from build123d import *

# Parameters (mm, degrees)
SKETCH1_W                         = 19.05
SKETCH1_H                         = 25.4
BOSS_EXTRUDE1_DEPTH               = 3.96875
SKETCH2_R                         = 9.921875
CUT_EXTRUDE1_DEPTH                = 24.236683855
SKETCH3_W                         = 7.14375
SKETCH3_H                         = 25.4
CUT_EXTRUDE2_DEPTH                = 24.236683855
SKETCH4_W                         = 6.35
SKETCH4_H                         = 9.525
BOSS_EXTRUDE2_DEPTH               = 7.14375
TAP_DRILL_FOR_2_HELICOIL1_D       = 2.38252
TAP_DRILL_FOR_2_HELICOIL3_D       = 2.38252
TAP_DRILL_FOR_2_HELICOIL3_DEPTH   = 4.7371
TAP_DRILL_FOR_2_HELICOIL3_TIP     = 0.715781221
TAP_DRILL_FOR_2_HELICOIL3_2_D     = 2.38252
TAP_DRILL_FOR_2_HELICOIL3_2_DEPTH = 4.7371
TAP_DRILL_FOR_2_HELICOIL3_2_TIP   = 0.715781221
FILLET1_R                         = 0.79375
FILLET2_RADIUS                    = 3.175
FILLET2_LENGTH                    = 9.525


with BuildPart() as part:
    # Sketch1 → Boss-Extrude1 (new body)
    with BuildSketch(Plane.XY):
        with Locations((9.525, 0)):
            Rectangle(SKETCH1_W, SKETCH1_H)
    extrude(amount=BOSS_EXTRUDE1_DEPTH)

    # Sketch2 → Cut-Extrude1 (cut, through all)
    with BuildSketch(Plane.XY.offset(3.96875)):
        Circle(SKETCH2_R)
    extrude(amount=-CUT_EXTRUDE1_DEPTH, mode=Mode.SUBTRACT)

    # Sketch3 → Cut-Extrude2 (cut, through all)
    with BuildSketch(Plane.XY.offset(3.96875)):
        with Locations((3.571875, 0)):
            Rectangle(SKETCH3_W, SKETCH3_H)
    extrude(amount=-CUT_EXTRUDE2_DEPTH, mode=Mode.SUBTRACT)

    # Sketch4 → Boss-Extrude2 (add)
    with BuildSketch(Plane.XY.offset(3.96875)):
        with Locations((15.875, 0)):
            Rectangle(SKETCH4_W, SKETCH4_H)
    extrude(amount=BOSS_EXTRUDE2_DEPTH)

    # Tap Drill for #2 Helicoil1 (through all)
    with Locations(Plane(origin=(0, 0, 0), x_dir=(-1, 0, 0), z_dir=(0, 0, -1))):
        with Locations((-9.779, 9.779), (-9.779, -9.779), (-15.875, 7.9375), (-15.875, -7.9375)):
            Hole(TAP_DRILL_FOR_2_HELICOIL1_D / 2)

    # Tap Drill for _2 Helicoil3
    with Locations(Plane(origin=(0, 4.7625, 0), x_dir=(1, 0, 0), z_dir=(0, 1, 0))):
        with Locations((15.875, -7.9375)):
            Hole(TAP_DRILL_FOR_2_HELICOIL3_D / 2, depth=TAP_DRILL_FOR_2_HELICOIL3_DEPTH)
            with Locations((0, 0, -(TAP_DRILL_FOR_2_HELICOIL3_DEPTH + TAP_DRILL_FOR_2_HELICOIL3_TIP / 2))):  # 118° drill point
                Cone(0, TAP_DRILL_FOR_2_HELICOIL3_D / 2, TAP_DRILL_FOR_2_HELICOIL3_TIP, mode=Mode.SUBTRACT)

    # Tap Drill for _2 Helicoil3 2
    with Locations(Plane(origin=(0, -4.7625, 0), x_dir=(-1, 0, 0), z_dir=(0, -1, 0))):
        with Locations((-15.875, -7.9375)):
            Hole(TAP_DRILL_FOR_2_HELICOIL3_2_D / 2, depth=TAP_DRILL_FOR_2_HELICOIL3_2_DEPTH)
            with Locations((0, 0, -(TAP_DRILL_FOR_2_HELICOIL3_2_DEPTH + TAP_DRILL_FOR_2_HELICOIL3_2_TIP / 2))):  # 118° drill point
                Cone(0, TAP_DRILL_FOR_2_HELICOIL3_2_D / 2, TAP_DRILL_FOR_2_HELICOIL3_2_TIP, mode=Mode.SUBTRACT)

    # Fillet1
    fillet1_edges = [part.edges().sort_by_distance(p)[0] for p in [
        (12.7, 0, 3.96875),
    ]]
    fillet(fillet1_edges, radius=FILLET1_R)

    # Fillet2: full round fillet: the end face becomes a half cylinder, R = half its width
    fillet2_face = Plane((15.875, 0, 11.1125), x_dir=(0, 1, 0), z_dir=(0, 0, 1))  # on the end face: x along it, z out of the body
    fillet2_slab = fillet2_face.offset(-FILLET2_RADIUS / 2) * Box(FILLET2_LENGTH, 2 * FILLET2_RADIUS, FILLET2_RADIUS, mode=Mode.PRIVATE)  # the body's end, R deep
    fillet2_round = Plane((15.875, 0, 7.9375), x_dir=(0, 0, 1), z_dir=(0, 1, 0)) * Cylinder(FILLET2_RADIUS, FILLET2_LENGTH, mode=Mode.PRIVATE)  # its axis R under the face
    add(fillet2_slab - fillet2_round, mode=Mode.SUBTRACT)


solid = part.part
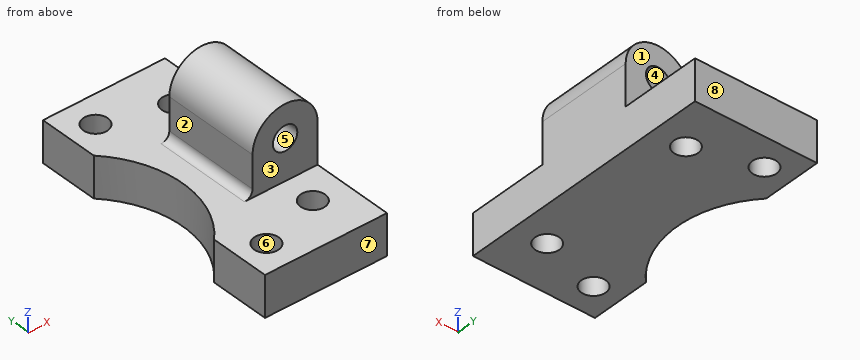
Could you check a few things on this model? Use its own coordinates, in mm. Face numbers are marked on the shaded views. A direction names the side the tool comes from. Coordinates: 2 decimals unless noted, no trailing zeros. Order: outer loops, then holes, each group sorted by start corner. A loop starts at its lowest first (then second) coordinate and runs counter-clockwise, first axis right, second up. Notation, with made-up numbers: (1, 3.25) - (27, 3.25) arc R24 cw to (27, 17.25) - close; hole circle Ø11 at (31.5, 32.5). An arc over 180 degrees is marked (long way). Answer in a Markdown table with one row per item. Add a question column.
(1) I need wall thicknesses on L1, parallel to Y at x = 12.75, z = 4.25; L2, parallel to Z at x = 15.75, y = 4.25; L3, parallel to Z at x = 10.5, y = 8.5. Which ranges of each line are inside material? Lowest first, please.
(2) If we section it at B-B, the plane x = 10.5: Please give me the cut outline in (y, z), then the cut area to 3 significant figures.
(3) Will these pins go through, and if not, where does the flat tip stop? pin 1 (6 mm diameter, centred on x = 12.5, y = 0, fed in from +Z); pin 2 (1.5 mm diameter, centred on y = -4.5, z = 5.5, fed in from -X); pin 3 (2 mm diameter, centred on x = 15.88, y = -7.94, fed in from +Z); pin 4 (2 mm diameter, centred on x = 14.5, z = 7.5, fed in from -Y).
(4) If we mould it in two halves opening along Y, with no side actions, what happens to the marked faces 5, 6, 7 and 8? For each: released by +Y, released by -Y, zero draft, split by the parting line, or undercut.
(5) On a 3-axis mill with a long thin cutter (end or side, diameter ignored), from which of +Z, -Z, +X, -X, +Y, -Y can I reach the whole of each face in a straight line? I mean the marked faces 1, 2, 3 and 4. Say none if no direction works.
(6) If we section it at D-D, the plane z = 3: State how many separate pieces and enclosed holes the cut face has, then the cut area to 3 significant figures.
(7) If we section it at A-A, the plane y = -7.5: Please give me the cut outline in (x, z), then the cut area to 3 significant figures.
Results are:
| question | item | result |
|---|---|---|
| 1 | L1 | y = -4.76 to 4.76 |
| 1 | L2 | z = 0 to 6.75, 9.12 to 11.11 |
| 1 | L3 | z = 0 to 3.97 |
| 2 | outline | (-12.7, 0) - (-10.73, 0) - (-10.73, 3.97) - (-12.7, 3.97) - close; (-8.83, 0) - (8.83, 0) - (8.83, 3.97) - (-8.83, 3.97) - close; (10.73, 0) - (12.7, 0) - (12.7, 3.97) - (10.73, 3.97) - close |
| 2 | area | 85.8 mm2 |
| 3 | pin 1 | stops at z = 11.09 |
| 3 | pin 2 | stops at x = 12.7 |
| 3 | pin 3 | passes through |
| 3 | pin 4 | stops at y = -4.76 |
| 4 | face 5 | zero draft |
| 4 | face 6 | undercut |
| 4 | face 7 | released by -Y |
| 4 | face 8 | released by +Y |
| 5 | face 1 | +Z, +X, -X, +Y |
| 5 | face 2 | +Z, -X, +Y, -Y |
| 5 | face 3 | +Z, +X, -X, -Y |
| 5 | face 4 | +Y |
| 6 | separate pieces | 1 |
| 6 | enclosed holes | 4 |
| 6 | area | 258 mm2 |
| 7 | outline | (7.14, 0) - (14.77, 0) - (14.77, 3.97) - (7.14, 3.97) - close; (16.98, 0) - (19.05, 0) - (19.05, 3.97) - (16.98, 3.97) - close |
| 7 | area | 38.5 mm2 |
